from build123d import *

# Parameters (mm, degrees)
SKETCH1_R                     = 5
SKETCH1_R_2                   = 1.5875
BOSS_EXTRUDE1_DEPTH           = 5
SKETCH2_R                     = 3.1
CUT_EXTRUDE1_DEPTH            = 5
CHAMFER1_SIZE                 = 0.5
M2_2X0_45_TAPPED_HOLE1_REACH  = 14.247
M2_2X0_45_TAPPED_HOLE1_BORE_R = 0.875


with BuildPart() as part:
    # Sketch1 → Boss-Extrude1 (new, symmetric)
    with BuildSketch(Plane.XY):
        Circle(SKETCH1_R)
        Circle(SKETCH1_R_2, mode=Mode.SUBTRACT)
    extrude(amount=BOSS_EXTRUDE1_DEPTH, both=True)

    # Sketch2 → Cut-Extrude1 (cut)
    with BuildSketch(Plane(origin=(0, 0, -5), x_dir=(-1, 0, 0), z_dir=(0, 0, -1))):
        Circle(SKETCH2_R)
    extrude(amount=-CUT_EXTRUDE1_DEPTH, mode=Mode.SUBTRACT)

    # Chamfer1
    chamfer1_edges = [part.edges().sort_by_distance(p)[0] for p in [
        (-5, 0, -5),
        (-5, 0, 5),
    ]]
    chamfer(chamfer1_edges, length=CHAMFER1_SIZE)

    # M2.2x0.45 Tapped Hole1 bore → M2.2x0.45 Tapped Hole1 (cut, up to next)
    with BuildSketch(Plane(origin=(0, -5, 0), x_dir=(-1, 0, 0), z_dir=(0, -1, 0)), mode=Mode.PRIVATE) as m2_2x0_45_tapped_hole1_sk1:
        with Locations((0, -3)):
            Circle(M2_2X0_45_TAPPED_HOLE1_BORE_R)
    m2_2x0_45_tapped_hole1_tool1 = extrude(m2_2x0_45_tapped_hole1_sk1.sketch, amount=-M2_2X0_45_TAPPED_HOLE1_REACH, mode=Mode.PRIVATE) & part.part
    # M2.2x0.45 Tapped Hole1 bore → M2.2x0.45 Tapped Hole1 (cut, up to next)
    with BuildSketch(Plane(origin=(0, -5, 0), x_dir=(-1, 0, 0), z_dir=(0, -1, 0)), mode=Mode.PRIVATE) as m2_2x0_45_tapped_hole1_sk2:
        with Locations((0, 3)):
            Circle(M2_2X0_45_TAPPED_HOLE1_BORE_R)
    m2_2x0_45_tapped_hole1_tool2 = extrude(m2_2x0_45_tapped_hole1_sk2.sketch, amount=-M2_2X0_45_TAPPED_HOLE1_REACH, mode=Mode.PRIVATE) & part.part
    add(m2_2x0_45_tapped_hole1_tool1.solids().sort_by_distance((0, -5, 3))[0], mode=Mode.SUBTRACT)
    add(m2_2x0_45_tapped_hole1_tool2.solids().sort_by_distance((0, -5, -3))[0], mode=Mode.SUBTRACT)


solid = part.part
Design review of the part built by this model. Coordinates are the model's own, in mm. A direction names the side the tool comes from. Coordinates: 2 decimals unless noted, no trailing zeros. Order: outer loops, then holes, each group sorted by start corner. A loop starts at its lowest first (then second) coordinate and runs counter-clockwise, first axis right, second up. Notation, with made-up numbers: (21, 62.25) -> (29, 62.25) arc R34 cw to (29, 99.25) -> close; hole circle Ø8 at (62.5, 87.25). An arc over 180 degrees is marked (long way). Use one line per item in the form item = value. Start each with the question number.
(1) Add section A-A on x = 0. State the section outline as (y, z) points (1 decimal), plus the area to 3 significant figures.
(2) Insertion check: pin 1 (4 mm diameter, centred on x = 0, y = 0, fed in from -Z); pin 2 (1.5 mm diameter, centred on x = 4, z = 1, fed in from +Y); pin 3 (3 mm diameter, centred on x = -3.5, z = 3.5, fed in from +Y). Each pin has a flat end and moves straight along its axis. Give the tip position at first contact, or say it passes through.
(3) Add section C-C on y = -4. Give the number of separate pieces and of enclosed holes in the cut face, plus the area to 3 significant figures.
(4) For faces 4 (the cylindrical face through (0.19, -4.001, -2.146)), 5 (the flat face through (0, -2, 5)), 6 (the flat face through (-1.3, -1.3, 0)), list the 3-axis set-ups (+Z, -Z, +X, -X, +Y, -Y) from which the entire face can be reached by the end or side of a thin tool; tool diameter is ignored.
(5) The part is to be moulded in two halves that separate along X. For faces 1 (the cylindrical face through (-1.67, 2.61, -2.54)), 2 (the cylindrical face through (-1.08, -4.88, 0.06)), 3 (the flat face through (-1.1, 3.1, -5)), say which applies: +X half, -X half, draft (parallel to the pull), parting line (faces both ways), or undercut.
(6) Add section B-B on z = 1. State the section outline as (x, y) points (1 decimal), plus the area to 3 significant figures.
(7) Add section D-D on z = 3. State the section outline as (x, y) points (1 decimal).
(8) For probe 1 along Z at (x, y) = (0, -4.3) (3 decimals); probe 2 along Y at (x, z) = (0, 3.7); probe 3 along Y at (x, z) = (1, -3.25), list the stretches that pass through material, from the lowest coordinate up.
Answer block:
q1.outline = (-5, -4.5) -> (-4.5, -5) -> (-3.1, -5) -> (-3.1, -3.9) -> (-5, -3.9) -> close; (-5, -2.1) -> (-3.1, -2.1) -> (-3.1, 0) -> (-1.6, 0) -> (-1.6, 2.1) -> (-5, 2.1) -> close; (-5, 3.9) -> (-1.6, 3.9) -> (-1.6, 5) -> (-4.5, 5) -> (-5, 4.5) -> close; (1.6, 0) -> (3.1, 0) -> (3.1, -5) -> (4.5, -5) -> (5, -4.5) -> (5, 4.5) -> (4.5, 5) -> (1.6, 5) -> close
q1.area = 43.3 mm²
q2.pin_1 = 0
q2.pin_2 = 3.8
q2.pin_3 = 4.58
q3.separate_pieces = 1
q3.enclosed_holes = 2
q3.area = 54.3 mm²
q4.face_4 = -Y
q4.face_5 = +Z, +X, -X, +Y, -Y
q4.face_6 = -Z
q5.face_1 = undercut
q5.face_2 = parting line
q5.face_3 = draft
q6.outline = circle Ø10 at (0, 0); hole circle Ø3.2 at (0, 0)
q6.area = 70.6 mm²
q7.outline = (-0.9, -4.9) -> (-0.9, -1.3) arc R1.6 cw (long way) to (0.9, -1.3) -> (0.9, -4.9) arc R5 ccw (long way) to start
q8.probe_1 = -5 to -3.875, -2.125 to 2.125, 3.875 to 5
q8.probe_2 = 1.59 to 5
q8.probe_3 = -4.9 to -2.93, 2.93 to 4.9
